Check sheet for the drawn part. Datum: minimum x, y, z corner. Units: mm. A direction names the side the tool comes from. Round coordinates to 2 decimals unless told otherwise and drop trailing zeros. Write each loop counter-clockwise with the first axis right and the second up, starting at its lowest first coordinate (ties: lowest second). Pieces come first, ordered by that corner, then holes.
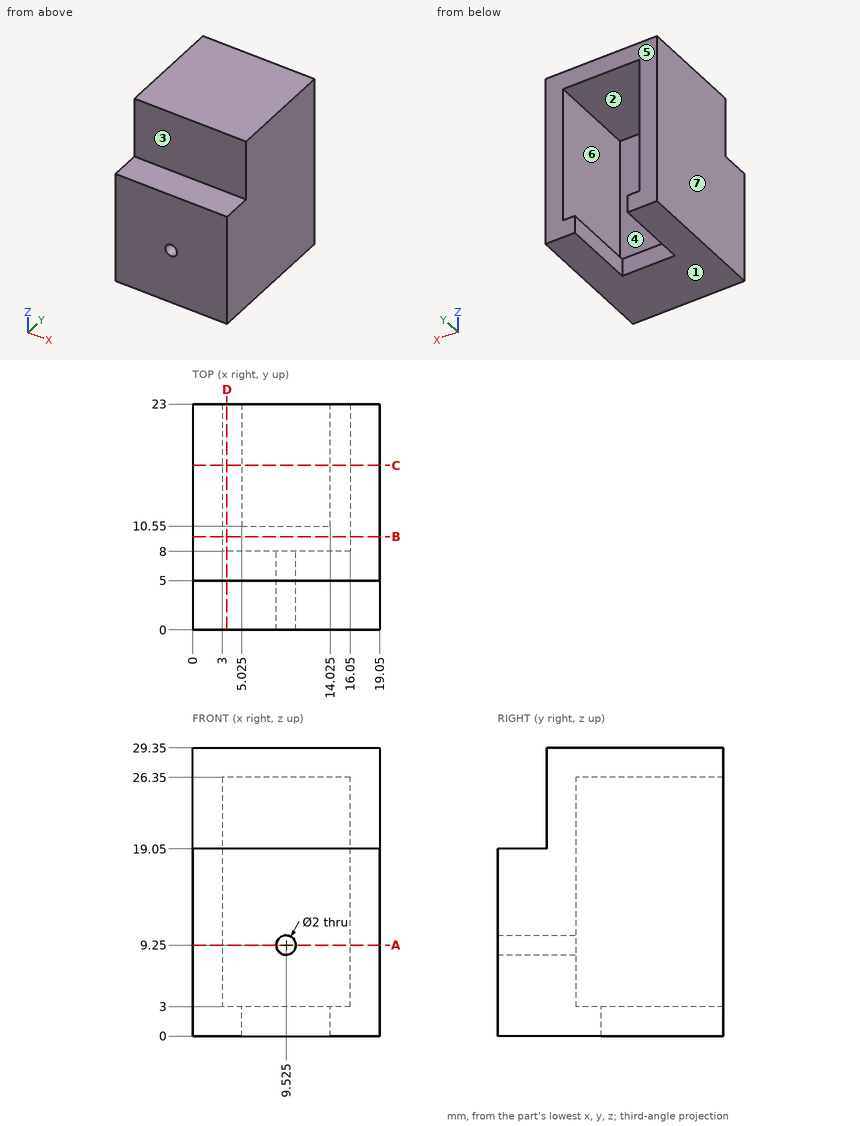
Q1. Sectioned sample at C-C (y = 16.75). Enter the section's corners in (x, z) (3 decimals), plus the area to 3 significant figures.
Recorded:
outline: (0, 0) - (5.025, 0) - (5.025, 3) - (3, 3) - (3, 26.35) - (16.05, 26.35) - (16.05, 3) - (14.025, 3) - (14.025, 0) - (19.05, 0) - (19.05, 29.35) - (0, 29.35) - close
area: 227 mm2
Q2. Sectioned sample at D-D (x = 3.5). Enter the section's corners in (y, z).
Recorded:
outline: (0, 0) - (23, 0) - (23, 3) - (8, 3) - (8, 26.35) - (23, 26.35) - (23, 29.35) - (5, 29.35) - (5, 19.05) - (0, 19.05) - close
Q3. Sectioned sample at B-B (y = 9.5). Enter the section's corners in (x, z), plus the area to 3 significant figures.
Recorded:
outline: (0, 0) - (19.05, 0) - (19.05, 29.35) - (0, 29.35) - close; hole (3, 3) - (16.05, 3) - (16.05, 26.35) - (3, 26.35) - close
area: 254 mm2
Q4. Sectioned sample at A-A (z = 9.25). Enter the section's corners in (x, y) (3 decimals), plus the area to 3 significant figures.
Recorded:
outline: (0, 0) - (8.525, 0) - (8.525, 8) - (3, 8) - (3, 23) - (0, 23) - close; (10.525, 0) - (19.05, 0) - (19.05, 23) - (16.05, 23) - (16.05, 8) - (10.525, 8) - close
area: 226 mm2
Q5. Release check for a two-part mould opening along X. For the marked faces 4, 5, 6 and 7 record: released by +X, released by -X, zero draft, split by the parting line, or undercut.
Recorded:
face 4: undercut
face 5: zero draft
face 6: undercut
face 7: released by -X
Q6. Depth check by flat-ended pin: P1, Ø4, axis at x = 9.5, z = 13.5, coming from the +Y side; P2, Ø0.9, axis at x = 9.5, z = 2, coming from the +Y side; P3, Ø5.5, axis at x = 13, y = 2, coming from the +Z side. Enter the tip coordinate at first touch or a pass-through.
Recorded:
P1: stops at y = 8
P2: stops at y = 10.55
P3: stops at z = 19.05
Q7. Tool access check on the marked faces 1, 2 and 3. Record the directions out of +Z, -Z, +X, -X, +Y, -Y that give a thin tool (end or side, any length) a straight path to the whole face; none if there is none.
Recorded:
face 1: -Z, +X, -X, +Y, -Y
face 2: +Y
face 3: +Z, +X, -X, -Y
Q8. Material ranges on line 1 along Z through (x, y) = (12.25, 9.75); line 2 along X through (y, z) = (1.75, 9.25) (3 decimals); line 3 along Y through (x, z) = (8.5, 5.25), recorded low to high.
Recorded:
line 1: z = 0 to 3, 26.35 to 29.35
line 2: x = 0 to 8.525, 10.525 to 19.05
line 3: y = 0 to 8
